CAD build for the part. Positions are in the model's coordinates, mm. A direction names the side the tool comes from. Coordinates: 2 decimals unless noted, no trailing zeros. Order: outer loops, then holes, each group sorted by start corner. A loop starts at its lowest first (then second) coordinate and runs counter-clockwise, first axis right, second up. Notation, with made-up numbers: (41, 71) - (95, 71) arc R4 cw to (95, 76) - close; hole circle Ø5 at (68.5, 85.5). An arc over 180 degrees is marked (long way). Write each question's results on one line, items separated by ' | '. Start each with the question number.
Q1. Which spindle directions (+Z, -Z, +X, -X, +Y, -Y) get a long thin tool onto all of the face, cutting with end or side? Do faces 1 (the flat face through (158, 1, -23)), 2 (the flat face through (84, 69, 0)), 3 (the flat face through (84, 0.737, -26)). Say none if no direction does.
Q2. Band-saw the part on A-A, the plane y = 18.5. Write the cut outline in (x, z).
Q3. Band-saw the part on C-C, the plane y = 94. Write the cut outline in (x, z), then the cut area to 3 significant figures.
Q4. Band-saw the part on D-D, the plane x = -24.5. Write the cut outline in (y, z), then the cut area to 3 significant figures.
Q5. Band-saw the part on B-B, the plane x = 7. Write the cut outline in (y, z).
Q6. Pin check, flat tips, straight feed: P1, Ø8, axis at x = -24.5, y = 94, coming from the -Z side; P2, Ø5, axis at x = 190, y = 53.94, coming from the +Z side; P3, Ø11.5, axis at x = 85.5, y = -33, coming from the -Z side; P4, Ø4, axis at y = 0.5, z = -15, coming from the -X side. Stop position of each tip, or through.
Q7. Wall check: probe 1 along Y at (x, z) = (195.5, -0.75); probe 2 along Y at (x, z) = (129.5, -23.5); probe 3 along Z at (x, y) = (163, 71). Give the ranges that are in metal, low to high.
```python
from build123d import *

# Parameters (mm, degrees)
SKETCH_1_W             = 271
SKETCH_1_H             = 167
SKETCH_1_R             = 2.25
SM_BASE_FLANGE_1_DEPTH = 1.2
SM_EDGE_FLANGE_1_DEPTH = 145
CUT_EXTRUDE_1_REACH    = 255.647
SKETCH_9_R             = 4.5


# Sheet-metal steps are written as plain solids
with BuildPart() as part:
    # Sketch 1 → Базовая кромка1 (new body)
    with BuildSketch(Plane.XY):
        with Locations((85.5, 30.5)):
            Rectangle(SKETCH_1_W, SKETCH_1_H)
        with Locations((176, 53.9366)):
            Circle(SKETCH_1_R, mode=Mode.SUBTRACT)
        with Locations((190, 53.9366)):
            Circle(SKETCH_1_R, mode=Mode.SUBTRACT)
        with Locations((165, -13.0634)):
            Circle(SKETCH_1_R, mode=Mode.SUBTRACT)
        with Locations((190, -13.0634)):
            Circle(SKETCH_1_R, mode=Mode.SUBTRACT)
        Polygon((13, 0), (158, 0), (158, -3), (171, -3), (171, 0), (171, 64), (0, 64), (0, 0), (0, -3), (13, -3), align=None, mode=Mode.SUBTRACT)
    extrude(amount=-SM_BASE_FLANGE_1_DEPTH)

    # Ребро-кромка1 section (across the edge) → Ребро-кромка1 (add)
    with BuildSketch(Plane(origin=(13, 0.7366, -1.2), x_dir=(0, -1, 0), z_dir=(1, 0, 0))):
        with BuildLine():
            Line((-1.2, 0.7366), (-1.2, 48.8))
            Line((-1.2, 48.8), (0, 48.8))
            Line((0, 48.8), (0, 0.7366))
            ThreePointArc((0, 0.7366), (0.215745145, 0.215745145), (0.7366, 0))
            Line((0.7366, 0), (0.7366, -1.2))
            ThreePointArc((0.7366, -1.2), (-0.632782992, -0.632782992), (-1.2, 0.7366))
        make_face()
    extrude(amount=SM_EDGE_FLANGE_1_DEPTH)

    # Эскиз9 → Вырез-Вытянуть1 (cut, up to next)
    with BuildSketch(Plane.XY, mode=Mode.PRIVATE) as cut_extrude_1_sk1:
        with Locations((-24.5, 94)):
            Circle(SKETCH_9_R)
    cut_extrude_1_tool1 = extrude(cut_extrude_1_sk1.sketch, amount=-CUT_EXTRUDE_1_REACH, mode=Mode.PRIVATE) & part.part
    # Эскиз9 → Вырез-Вытянуть1 (cut, up to next)
    with BuildSketch(Plane.XY, mode=Mode.PRIVATE) as cut_extrude_1_sk2:
        with Locations((-24.5, -33)):
            Circle(SKETCH_9_R)
    cut_extrude_1_tool2 = extrude(cut_extrude_1_sk2.sketch, amount=-CUT_EXTRUDE_1_REACH, mode=Mode.PRIVATE) & part.part
    # Эскиз9 → Вырез-Вытянуть1 (cut, up to next)
    with BuildSketch(Plane.XY, mode=Mode.PRIVATE) as cut_extrude_1_sk3:
        with Locations((85.5, -33)):
            Circle(SKETCH_9_R)
    cut_extrude_1_tool3 = extrude(cut_extrude_1_sk3.sketch, amount=-CUT_EXTRUDE_1_REACH, mode=Mode.PRIVATE) & part.part
    # Эскиз9 → Вырез-Вытянуть1 (cut, up to next)
    with BuildSketch(Plane.XY, mode=Mode.PRIVATE) as cut_extrude_1_sk4:
        with Locations((85.5, 94)):
            Circle(SKETCH_9_R)
    cut_extrude_1_tool4 = extrude(cut_extrude_1_sk4.sketch, amount=-CUT_EXTRUDE_1_REACH, mode=Mode.PRIVATE) & part.part
    # Эскиз9 → Вырез-Вытянуть1 (cut, up to next)
    with BuildSketch(Plane.XY, mode=Mode.PRIVATE) as cut_extrude_1_sk5:
        with Locations((195.5, 94)):
            Circle(SKETCH_9_R)
    cut_extrude_1_tool5 = extrude(cut_extrude_1_sk5.sketch, amount=-CUT_EXTRUDE_1_REACH, mode=Mode.PRIVATE) & part.part
    # Эскиз9 → Вырез-Вытянуть1 (cut, up to next)
    with BuildSketch(Plane.XY, mode=Mode.PRIVATE) as cut_extrude_1_sk6:
        with Locations((195.5, -33)):
            Circle(SKETCH_9_R)
    cut_extrude_1_tool6 = extrude(cut_extrude_1_sk6.sketch, amount=-CUT_EXTRUDE_1_REACH, mode=Mode.PRIVATE) & part.part
    add(cut_extrude_1_tool1.solids().sort_by_distance((-24.5, 94, 0))[0], mode=Mode.SUBTRACT)
    add(cut_extrude_1_tool2.solids().sort_by_distance((-24.5, -33, 0))[0], mode=Mode.SUBTRACT)
    add(cut_extrude_1_tool3.solids().sort_by_distance((85.5, -33, 0))[0], mode=Mode.SUBTRACT)
    add(cut_extrude_1_tool4.solids().sort_by_distance((85.5, 94, 0))[0], mode=Mode.SUBTRACT)
    add(cut_extrude_1_tool5.solids().sort_by_distance((195.5, 94, 0))[0], mode=Mode.SUBTRACT)
    add(cut_extrude_1_tool6.solids().sort_by_distance((195.5, -33, 0))[0], mode=Mode.SUBTRACT)


solid = part.part
```
Results below:
1) face 1: +Z, -Z | face 2: +Z, +X, -X, +Y, -Y | face 3: -Z, +X, -X, -Y
2) outline: (-50, -1.2) - (0, -1.2) - (0, 0) - (-50, 0) - close; (171, -1.2) - (221, -1.2) - (221, 0) - (171, 0) - close
3) outline: (-50, -1.2) - (-29, -1.2) - (-29, 0) - (-50, 0) - close; (-20, -1.2) - (81, -1.2) - (81, 0) - (-20, 0) - close; (90, -1.2) - (191, -1.2) - (191, 0) - (90, 0) - close; (200, -1.2) - (221, -1.2) - (221, 0) - (200, 0) - close | area: 293 mm²
4) outline: (-53, -1.2) - (-37.5, -1.2) - (-37.5, 0) - (-53, 0) - close; (-28.5, -1.2) - (89.5, -1.2) - (89.5, 0) - (-28.5, 0) - close; (98.5, -1.2) - (114, -1.2) - (114, 0) - (98.5, 0) - close | area: 179 mm²
5) outline: (-53, -1.2) - (-3, -1.2) - (-3, 0) - (-53, 0) - close; (64, -1.2) - (114, -1.2) - (114, 0) - (64, 0) - close
6) P1: passes through | P2: stops at z = 0 | P3: stops at z = -1.2 | P4: stops at x = 13
7) probe 1: y = -53 to -37.5, -28.5 to 89.5, 98.5 to 114 | probe 2: y = 0.74 to 1.94 | probe 3: z = -1.2 to 0
